from build123d import *

# Parameters (mm, degrees)
F0_W     = 60
F0_H     = 80
F0_R     = 2
F1_DEPTH = 30
F2_DEPTH = 32
F3_R     = 5


# Not quite as in the source:
# - a feature names something its author has since deleted; it is built from what else it names


with BuildPart() as f1:
    # F0 (on Front) → F1 (new body)
    with BuildSketch(Plane.XZ):
        Rectangle(F0_W, F0_H)
        with Locations((-15, -30.0458669662)):
            Circle(F0_R, mode=Mode.SUBTRACT)
        with Locations((-5, -30.0458669662)):
            Circle(F0_R, mode=Mode.SUBTRACT)
        with Locations((5, -30.0458669662)):
            Circle(F0_R, mode=Mode.SUBTRACT)
        with Locations((15, -30.3212571889)):
            Circle(F0_R, mode=Mode.SUBTRACT)
    extrude(amount=F1_DEPTH)

    # F0 (on Front) → F2 (join)
    with BuildSketch(Plane.XZ):
        with Locations((-15, -30.0458669662)):
            Circle(F0_R)
        with Locations((15, -30.3212571889)):
            Circle(F0_R)
        with Locations((-5, -30.0458669662)):
            Circle(F0_R)
        with Locations((5, -30.0458669662)):
            Circle(F0_R)
    extrude(amount=F2_DEPTH)

    # F3
    f3_edges = [f1.edges().sort_by_distance(p)[0] for p in [
        (0, -30, 40),
        (0, 0, 40),
        (30, -15, 40),
        (-30, -15, 40),
        (-30, -30, 0),
        (30, -30, 0),
        (-30, 0, 0),
        (30, 0, 0),
    ]]
    fillet(f3_edges, radius=F3_R)


solid = f1.part
Part model, mm, in its own coordinate system. A direction names the side the tool comes from. Round coordinates to 2 decimals unless told otherwise and drop trailing zeros. Write each loop counter-clockwise with the first axis right and the second up, starting at its lowest first coordinate (ties: lowest second). Pieces come first, ordered by that corner, then holes. Notation, with made-up numbers: (11.5, -2) - (29.5, -2) arc R22 cw to (29.5, 20) - close; hole circle Ø3 at (73, -8). An arc over 180 degrees is marked (long way). Use CSV: the item, a comma, the result in double quotes.
Item 1: Flat gauge pins, fed straight in: P1, Ø1, axis at x = -5.5, y = -4, coming from the +Z side; P2, Ø2, axis at x = -18, z = 19.5, coming from the -Y side; P3, Ø2, axis at y = -28, z = 1, coming from the +X side. Where does each tip first touch, or does it go through?
Results list:
P1,"stops at z = 39.97"
P2,"stops at y = -30"
P3,"stops at x = 29.58"
Item 2: Slice it at C-C, the plane y = -2.5. Write the cut outline in (x, z), then the cut area to 3 significant figures.
Results list:
outline,"(-29.33, -40) - (29.33, -40) - (29.33, 35) arc R4.33 ccw to (25, 39.33) - (-25, 39.33) arc R4.33 ccw to (-29.33, 35) - close"
area,"4,650 mm²"
Item 3: Wall check: L1, parallel to Y at x = -4, z = -25.5; L2, parallel to X at y = -3.5, z = -19; L3, parallel to Z at x = 18, y = -1.5. Give the ranges that are in metal, low to high.
Results list:
L1,"y = -30 to 0"
L2,"x = -29.77 to 29.77"
L3,"z = -40 to 38.57"
Item 4: Slice it at B-B, the plane x = -5. Write the cut outline in (y, z), then the cut area to 3 significant figures.
Results list:
outline,"(-32, -32.05) - (-30, -32.05) - (-30, -40) - (0, -40) - (0, 35) arc R5 ccw to (-5, 40) - (-25, 40) arc R5 ccw to (-30, 35) - (-30, -28.05) - (-32, -28.05) - close"
area,"2,400 mm²"
Item 5: Tool access for faces 5 (the flat face through (0, -15, -40)), 6 (the cylindrical face through (4.74, -30.986, -28.063)): list every direction of +Z, -Z, +X, -X, +Y, -Y with a clear straight run to the whole face (end or side of a thin tool).
Results list:
face 5,"-Z, +X, -X, +Y, -Y"
face 6,"-Y"
Item 6: Slice it at A-A, the plane z = -22.5. Write the cut outline in (x, y).
Results list:
outline,"(-30, -25) arc R5 ccw to (-25, -30) - (25, -30) arc R5 ccw to (30, -25) - (30, -5) arc R5 ccw to (25, 0) - (-25, 0) arc R5 ccw to (-30, -5) - close"
Item 7: Pull direction X, two halves, no side cores. Call faces 1 (the flat face through (-5, -32, -30)), 2 (the flat face through (-30, -15, -3)), 3 (the cylindrical face through (-15.26, -30.986, -28.063)), 4 (the cylindrical face through (-5.26, -30.986, -28.063)): pulls with the +X half, pulls with the -X half, needs draft (parallel to the pull), parting line crosses it, or undercut.
Results list:
face 1,"needs draft"
face 2,"pulls with the -X half"
face 3,"undercut"
face 4,"undercut"
